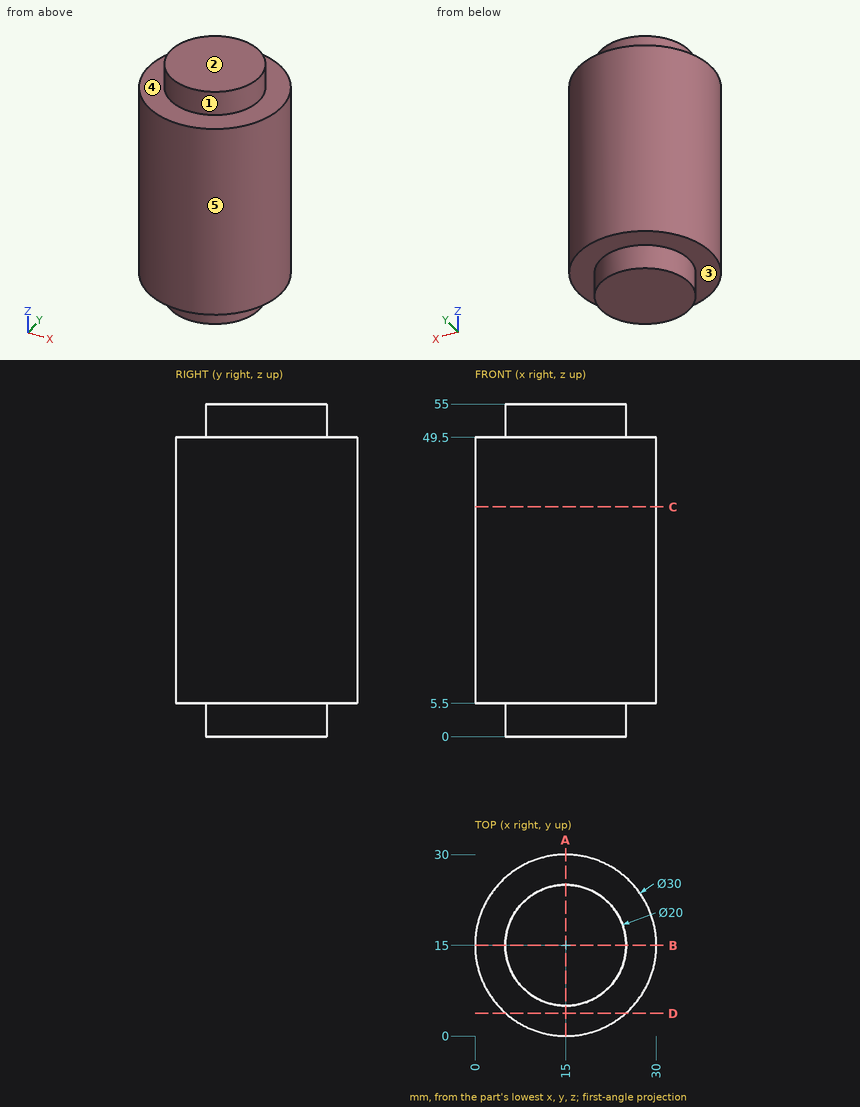
The figure shows three views and two pictorial views of one solid part (mm, origin at its lowest corner). Answer the questions. A direction names the side the tool comes from. Coordinates: 2 decimals unless noted, no trailing zeros. Order: outer loops, then holes, each group sorted by start corner. A loop starts at its lowest first (then second) coordinate and runs counter-clockwise, first axis right, second up.
Q1. For a pull along Y with two mould halves and no side action, classify the marked faces 4 and 5 as pulls with the +Y half, pulls with the -Y half, needs draft (parallel to the pull), parting line crosses it, or undercut.
Q2. Consider line 1 (Z direction, x = 5.5, y = 11.5); line 2 (Y direction, x = 14.75, z = 3); line 3 (X direction, y = 18.25, z = 20.5). Determine where each line is inside the solid, lowest interval first.
Q3. A cutting plane is placed at C-C, the plane z = 38. Write down the section's boundary in (x, y), and give its area (3 significant figures).
Q4. Given P1, Ø10, axis at x = 14, y = 11, coming from the -Z side; P2, Ø6, axis at y = 19.5, z = 47, coming from the +X side; P3, Ø8, axis at y = 25, z = 38.5, coming from the +X side, each flat-ended and moving along its own axis, determine where each tip first touches the part or whether it passes through.
Q5. A cutting plane is placed at D-D, the plane y = 3.75. Write down the section's boundary in (x, z).
Q6. Which of the six approach directions +Z, -Z, +X, -X, +Y, -Y give full straight-line access (tool end or side, diameter ignored) to the marked faces 1, 2 and 3?
Q7. A cutting plane is placed at A-A, the plane x = 15. Write down the section's boundary in (y, z), and give its area (3 significant figures).
Answers follow:
1. face 4: needs draft
1. face 5: parting line crosses it
2. line 1: z = 5.5 to 49.5
2. line 2: y = 5 to 25
2. line 3: x = 0.36 to 29.64
3. outline: circle Ø30 at (15, 15)
3. area: 707 mm2
4. P1: stops at z = 0
4. P2: stops at x = 29.92
4. P3: stops at x = 28.75
5. outline: (5.08, 5.5) - (24.92, 5.5) - (24.92, 49.5) - (5.08, 49.5) - close
6. face 1: +Z
6. face 2: +Z, +X, -X, +Y, -Y
6. face 3: -Z
7. outline: (0, 5.5) - (5, 5.5) - (5, 0) - (25, 0) - (25, 5.5) - (30, 5.5) - (30, 49.5) - (25, 49.5) - (25, 55) - (5, 55) - (5, 49.5) - (0, 49.5) - close
7. area: 1,540 mm2
